Geometry: see drawing. Coordinates: mm, zero at the bounding-box minimum. A direction names the side the tool comes from. Give positions to 0.01 mm unless a question says otherwise; leave off trailing zeros. Write each loop counter-clockwise with the first axis right and the second up, starting at its lowest first coordinate (ties: lowest second). Pieces come first, ordered by that corner, then holes. Notation, with made-up numbers: M 52.5,0.25 L 56.5,0.25 A23 ccw 56.5,36.25 Z; hole C 54,8.5 d8. An arc over 180 degrees is marked long. Use one line per item in the form item = value. Start each with the question number.
Item 1: Section query D-D on x = 20. Return loops of the section in (y, z), then the cut area to 3 significant figures.
Item 2: Pull-direction query (Y, two-part tool) for the marked faces 4, 5, 6 and 7; classes: released by +Y, released by -Y, zero draft, split by the parting line, or undercut.
Item 3: Access query for the marked faces 1, 2 and 3. Directions: +Z, -Z, +X, -X, +Y, -Y. A direction counts if a zero-diameter tool reaches every point of the face in a straight line with its end or side. Return the directions, or none.
Item 4: Section query A-A on x = 35. Return loops of the section in (y, z), then the cut area to 3 significant figures.
Item 5: Contact query for flat-ended pins moving along their axis: P1, Ø2, axis at x = 12.5, z = 48, coming from the +Y side; P2, Ø6, axis at x = 25, y = 10, coming from the +Z side; P3, Ø8.5, axis at x = 50, z = 13.5, coming from the -Y side; P4, Ø1, axis at x = 10, y = 3.5, coming from the +Z side. Output: stop coordinate, or through.
Item 6: Section query C-C on z = 16. Return loops of the section in (x, y).
Item 7: Material intervals for line 1 along X through (y, z) = (24, 16); line 2 along Y through (x, z) = (36.25, 46); line 3 along Z through (x, y) = (55, 16.5), sorted ascending. Write a range as from..to.
Item 8: Section query B-B on y = 23. Return loops of the section in (x, z).
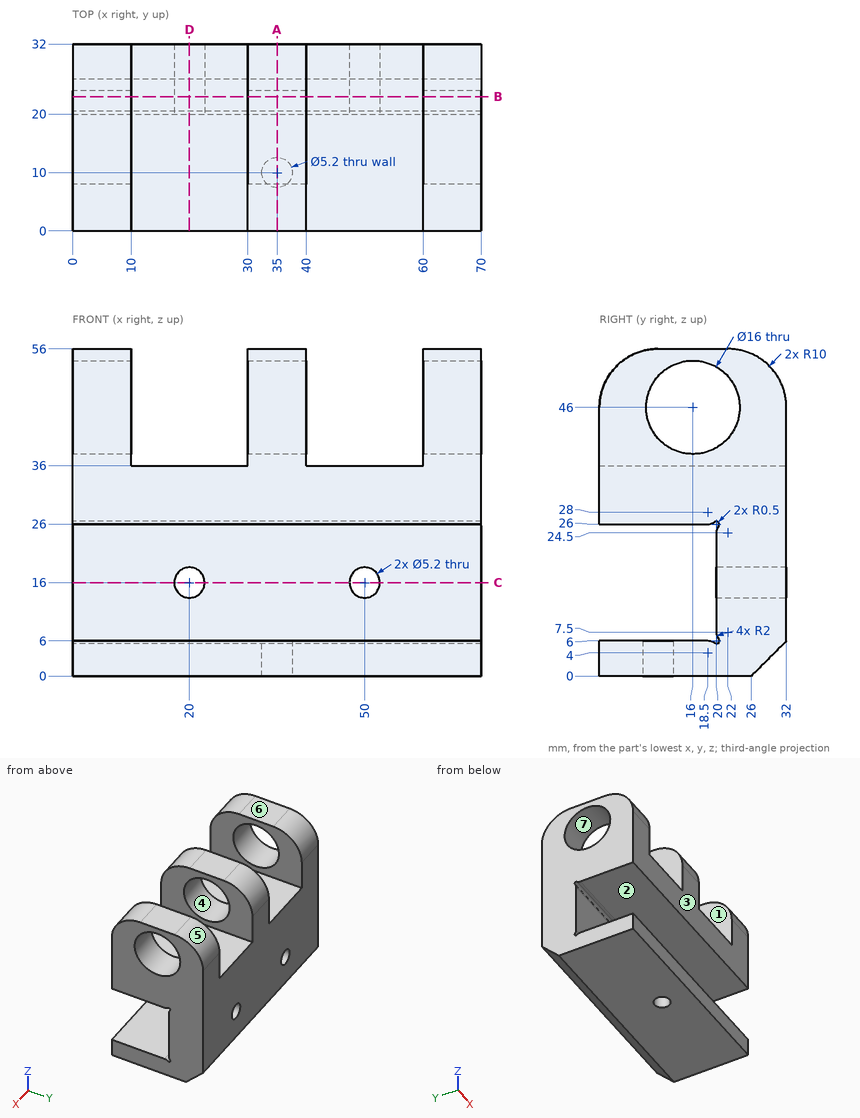
Answer sheet:
q1.outline = M 0,0 L 26,0 L 32,6 L 32,13.4 L 20,13.4 L 20,7.5 A2 ccw 20.4,6.3 A0.5 cw 19.7,5.6 A2 ccw 18.5,6 L 0,6 Z; M 0,26 L 18.5,26 A2 ccw 19.7,26.4 A0.5 cw 20.4,25.7 A2 ccw 20,24.5 L 20,18.6 L 32,18.6 L 32,36 L 0,36 Z
q1.area = 670 mm2
q2.face_4 = undercut
q2.face_5 = released by +Y
q2.face_6 = zero draft
q2.face_7 = undercut
q3.face_1 = +Z, +Y, -Y
q3.face_2 = +X, -X, -Y
q3.face_3 = +Z, -Z, +X, -X, -Y
q4.outline = M 0,0 L 7.4,0 L 7.4,6 L 0,6 Z; M 0,26 L 18.5,26 A2 ccw 19.7,26.4 A0.5 cw 20.4,25.7 A2 ccw 20,24.5 L 20,7.5 A2 ccw 20.4,6.3 A0.5 cw 19.7,5.6 A2 ccw 18.5,6 L 12.6,6 L 12.6,0 L 26,0 L 32,6 L 32,46 A10 ccw 22,56 L 10,56 A10 ccw 0,46 Z; hole C 16,46 d16
q4.area = 1,100 mm2
q5.P1 = through
q5.P2 = 36
q5.P3 = 20
q5.P4 = 54
q6.outline = M 0,20 L 17.4,20 L 17.4,32 L 0,32 Z; M 22.6,20 L 47.4,20 L 47.4,32 L 22.6,32 Z; M 52.6,20 L 70,20 L 70,32 L 52.6,32 Z
q7.line_1 = 0..17.4, 22.6..47.4, 52.6..70
q7.line_2 = 0..8, 24..32
q7.line_3 = 0..6, 26..36
q8.outline = M 0,0 L 70,0 L 70,42.13 L 60,42.13 L 60,36 L 40,36 L 40,42.13 L 30,42.13 L 30,36 L 10,36 L 10,42.13 L 0,42.13 Z; M 0,49.87 L 10,49.87 L 10,55.95 L 0,55.95 Z; M 30,49.87 L 40,49.87 L 40,55.95 L 30,55.95 Z; M 60,49.87 L 70,49.87 L 70,55.95 L 60,55.95 Z; hole C 20,16 d5.2; hole C 50,16 d5.2
